Autodesk Inventor part; units mm, degrees
ref_plane "YZ Plane" through (0, 0, 0) normal (1, 0, 0) x (0, 1, 0)
ref_plane "XZ Plane" through (0, 0, 0) normal (0, 1, 0) x (-1, 0, 0)
ref_plane "XY Plane" through (0, 0, 0) normal (0, 0, 1) x (1, 0, 0)
sketch "Sketch1" plane through (0, 0, 0) normal (0, 1, 0) x (-1, 0, 0)
  line L0 (0, 0) -> (-34.29, 0)
  line L1 (-34.29, 0) -> (-34.29, 25.4)
  line L2 (-34.29, 25.4) -> (0, 25.4)
  line L3 (0, 25.4) -> (0, 0)
  line L4 (0, 25.4) -> (-2.54, 25.4) construction
  line L5 (-2.54, 25.4) -> (-2.54, 22.86) construction
  line L6 (-2.54, 22.86) -> (0, 22.86) construction
  line L7 (0, 22.86) -> (0, 25.4) construction
  line L8 (0, 0) -> (-2.54, 0) construction
  line L9 (-2.54, 0) -> (-2.54, 2.54) construction
  line L10 (-2.54, 2.54) -> (0, 2.54) construction
  line L11 (0, 2.54) -> (0, 0) construction
  line L12 (-34.29, 25.4) -> (-31.75, 25.4) construction
  line L13 (-31.75, 25.4) -> (-31.75, 22.86) construction
  line L14 (-31.75, 22.86) -> (-34.29, 22.86) construction
  line L15 (-34.29, 22.86) -> (-34.29, 25.4) construction
  line L16 (-34.29, 0) -> (-31.75, 0) construction
  line L17 (-31.75, 0) -> (-31.75, 2.54) construction
  line L18 (-31.75, 2.54) -> (-34.29, 2.54) construction
  line L19 (-34.29, 2.54) -> (-34.29, 0) construction
  circle A0 centre (-2.54, 22.86) radius 1.0922
  circle A1 centre (-2.54, 2.54) radius 1.0922
  circle A2 centre (-31.75, 2.54) radius 1.0922
  circle A3 centre (-31.75, 22.86) radius 1.0922
  line L20 (0.635, 26.035) -> (-34.925, 26.035)
  line L21 (-34.925, 26.035) -> (-34.925, -0.635)
  line L22 (-34.925, -0.635) -> (0.635, -0.635)
  line L23 (0.635, -0.635) -> (0.635, 26.035)
  dimension "d0" = 34.29
  dimension "d1" = 25.4
  dimension "d2" = 2.54
  dimension "d3" = 2.54
  dimension "d4" = 2.54
  dimension "d5" = 2.54
  dimension "d6" = 2.54
  dimension "d7" = 2.54
  dimension "d8" = 2.54
  dimension "d9" = 2.54
  dimension "d10" = 2.1844
  dimension "d11" = 2.1844
  dimension "d12" = 2.1844
  dimension "d13" = 2.1844
  dimension "d14" = 0.635
extrude "Extrusion1" add sketch "Sketch1" along normal blind 3.175 contours L0 L1 L2 L3 | L23 L22 L21 L20
sketch "Sketch2" plane through (0, 3.175, 0) normal (0, 1, 0) x (1, 0, 0)
  line L0 (34.925, -26.035) -> (34.925, 0.635)
  line L1 (34.925, 0.635) -> (-0.635, 0.635)
  line L2 (-0.635, 0.635) -> (-0.635, -26.035)
  line L3 (-0.635, -26.035) -> (34.925, -26.035)
  circle A0 centre (2.54, -22.86) radius 1.0922
  circle A1 centre (2.54, -2.54) radius 1.0922
  circle A2 centre (31.75, -2.54) radius 1.0922
  circle A3 centre (31.75, -22.86) radius 1.0922
  line L4 (-3.81, -29.21) -> (-3.81, 3.81)
  line L5 (-3.81, 3.81) -> (38.1, 3.81)
  line L6 (38.1, 3.81) -> (38.1, -29.21)
  line L7 (38.1, -29.21) -> (-3.81, -29.21)
  point P0 (0, 0)
  dimension "d17" = 3.175
extrude "Extrusion2" add sketch "Sketch2" along normal blind 24 and the other way blind 3.175 contours L4 L5 L6 L7
sketch "Sketch3" plane through (38.1, 0, -3.81) normal (1, 0, 0) x (0, 0, -1)
  line L0 (-3.175, 27.175) -> (-29.845, 27.175)
  line L1 (-16.51, 27.175) -> (-24.01, 27.175)
  line L2 (-24.01, 27.175) -> (-9.01, 27.175)
  line L3 (-9.01, 27.175) -> (-9.01, 3.175)
  line L4 (-29.845, 3.175) -> (-3.175, 3.175)
  line L5 (-24.01, 27.175) -> (-24.01, 3.175)
  point P0 (-3.81, 0)
  dimension "d22" = 7.5
  dimension "d23" = 15
extrude "Extrusion3" cut sketch "Sketch3" against normal blind 24
sketch "Sketch4" plane through (-0.635, 3.175, 26.035) normal (1, 0, 0) x (0, 0, -1)
  line L0 (29.845, 24) -> (-3.175, 24)
  line L1 (13.335, 24) -> (6.835, 24)
  line L2 (6.835, 24) -> (19.835, 24)
  line L3 (26.67, 0) -> (0, 0)
  line L4 (19.835, 24) -> (6.835, 24)
  line L5 (6.835, 24) -> (6.835, 0)
  line L6 (6.835, 0) -> (19.835, 0)
  line L7 (19.835, 0) -> (19.835, 24)
  point P0 (26.035, -3.175)
  dimension "d26" = 6.5
  dimension "d27" = 13
extrude "Extrusion4" cut sketch "Sketch4" against normal blind 24
sketch "Sketch5" plane through (0, 0, 0) normal (0, -1, 0) x (1, 0, 0)
  line L0 (38.1, -3.81) -> (38.1, 29.21)
  line L1 (38.1, 29.21) -> (-3.81, 29.21)
  line L2 (-3.81, 29.21) -> (-3.81, -3.81)
  line L3 (-3.81, -3.81) -> (38.1, -3.81)
  circle A0 centre (2.54, 22.86) radius 1.0922
  circle A1 centre (2.54, 2.54) radius 1.0922
  circle A2 centre (31.75, 2.54) radius 1.0922
  circle A3 centre (31.75, 22.86) radius 1.0922
  line L4 (-0.635, -0.635) -> (-0.635, 26.035)
  line L5 (-0.635, 26.035) -> (34.925, 26.035)
  line L6 (34.925, 26.035) -> (34.925, -0.635)
  line L7 (34.925, -0.635) -> (-0.635, -0.635)
  line L8 (17.145, 29.21) -> (17.145, 35.56)
  line L9 (17.145, -3.81) -> (17.145, -10.16)
  circle A4 centre (17.145, 35.56) radius 2
  circle A5 centre (17.145, -10.16) radius 2
  circle A6 centre (17.145, 35.56) radius 6.35
  circle A7 centre (17.145, -10.16) radius 6.35
  line L10 (23.495, 35.56) -> (23.495, 29.21)
  line L11 (10.795, 35.56) -> (10.795, 29.21)
  line L12 (10.795, -10.16) -> (10.795, -3.81)
  line L13 (23.495, -10.16) -> (23.495, -3.81)
  point P0 (0, 0)
  dimension "d30" = 3.175
  dimension "d31" = 6.35
  dimension "d32" = 6.35
  dimension "d33" = 4
  dimension "d34" = 4
extrude "Extrusion5" add sketch "Sketch5" along normal blind 6.35 contours L3 L2 L1 L0 | L13 A7 L3 | L1 A6 L10 | A7 L12 L3 | A7 | L1 L11 A6 | A6
sketch "Sketch6" plane through (0, 3.175, 0) normal (0, 1, 0) x (1, 0, 0)
  circle A0 centre (31.75, -22.86) radius 1.0922
  circle A1 centre (31.75, -2.54) radius 1.0922
  circle A2 centre (2.54, -2.54) radius 1.0922
  circle A3 centre (2.54, -22.86) radius 1.0922
  line L0 (34.925, -5.2) -> (34.925, 0.635)
  line L1 (34.925, 0.635) -> (-0.635, 0.635)
  line L2 (-0.635, 0.635) -> (-0.635, -6.2)
  line L3 (-0.635, -6.2) -> (-3.81, -6.2)
  line L4 (-3.81, -19.2) -> (-3.81, -6.2)
  line L5 (-0.635, -19.2) -> (-3.81, -19.2)
  line L6 (-0.635, -19.2) -> (-0.635, -26.035)
  line L7 (-0.635, -26.035) -> (34.925, -26.035)
  line L8 (34.925, -26.035) -> (34.925, -20.2)
  line L9 (38.1, -20.2) -> (34.925, -20.2)
  line L10 (38.1, -5.2) -> (38.1, -20.2)
  line L11 (38.1, -5.2) -> (34.925, -5.2)
  line L12 (-0.635, -6.2) -> (-0.635, -19.2)
  line L13 (34.925, -5.2) -> (34.925, -20.2)
  point P0 (0, 0)
extrude "Extrusion6" add sketch "Sketch6" along normal blind 4 contours L11 L10 L9 L13 | L12 L5 L4 L3
sketch "Sketch7" plane through (0, 0, 0) normal (0, 1, 0) x (1, 0, 0)
  line L0 (10.795, 3.81) -> (23.495, 3.81)
  line L1 (23.495, 10.16) -> (23.495, 3.81)
  arc A0 (23.495, 10.16) -> (10.795, 10.16) centre (17.145, 10.16) ccw
  line L2 (10.795, 3.81) -> (10.795, 10.16)
  circle A1 centre (17.145, 10.16) radius 2
  circle A2 centre (17.145, -35.56) radius 2
  line L3 (23.495, -29.21) -> (10.795, -29.21)
  line L4 (10.795, -35.56) -> (10.795, -29.21)
  arc A3 (10.795, -35.56) -> (23.495, -35.56) centre (17.145, -35.56) ccw
  line L5 (23.495, -29.21) -> (23.495, -35.56)
  point P0 (0, 0)
extrude "Extrusion7" cut sketch "Sketch7" against normal blind 3.175
properties part number "pololuCaseBottom"
The listing builds one solid part. Answer for the finished solid, in the listing's coordinates (mm). A direction names the side the tool comes from. Round coordinates to 2 decimals unless told otherwise and drop trailing zeros. Loops run counter-clockwise (first coordinate to the right, second up) from the corner with the lowest first, then second, coordinate; pieces in that order, holes last.
Q1. Find the intervals of material crossed by line 1 (Z direction, x = 6, y = 15.5) (3 decimals); line 2 (X direction, y = 11, z = 4) (3 decimals); line 3 (X direction, y = 2, z = 22), in increasing order.
Q2. Section A-A, the plane x = 2.54 is taken. Determine the outline of the cut face in (y, z) (3 decimals).
Q3. Which of the six approach directions +Z, -Z, +X, -X, +Y, -Y give full straight-line access (tool end or side, diameter ignored) to faces 1 (the face through (-2, 17, 19.2)), 2 (the face through (17, 15, 26.035)), 3 (the face through (23.495, -5, -7)), 4 (the face through (17, -3, -0.635))?
Q4. Section D-D, the plane x = 8.5 is taken. Determine the outline of the cut face in (y, z) (3 decimals).
Q5. For a pull along X with two mould halves and no side action, classify faces 5 (the face through (17, 0, 13)), 6 (the face through (10.795, -5, 32)), 7 (the face through (37, 17, 20.2)), 8 (the face through (38.1, 6, 12)) as released by +X, released by -X, zero draft, split by the parting line, or undercut.
Q6. Section C-C, the plane y = 5 is taken. Determine the outline of the cut face in (x, z) (3 decimals), then the cut area to 3 significant figures.
Q7. Given pin 1 Ø3.5 at (x, y) = (37, 17.5) entering from +Z; pin 2 Ø2 at (x, z) = (11.5, 18.5) entering from -Y; pin 3 Ø3.5 at (y, z) = (-5, 33) entering from +X (3 decimals), each flat-ended and moving along its own axis, determine where each tip first touches the part or whether it passes through.
Q8. Section B-B, the plane z = 0.5 is taken. Determine the outline of the cut face in (x, y) (3 decimals), then the cut area to 3 significant figures.
Completed:
1. line 1: z = -3.81 to -0.635, 26.035 to 29.21
1. line 2: x = -3.81 to -0.635, 34.925 to 38.1
1. line 3: x = -3.81 to 1.87, 3.21 to 31.08, 32.42 to 38.1
2. outline: (-6.35, -3.81) - (27.175, -3.81) - (27.175, -0.635) - (3.175, -0.635) - (3.175, 1.448) - (0, 1.448) - (0, -0.635) - (-6.35, -0.635) - close; (-6.35, 26.035) - (0, 26.035) - (0, 23.952) - (3.175, 23.952) - (3.175, 26.035) - (27.175, 26.035) - (27.175, 29.21) - (-6.35, 29.21) - close; (0, 3.632) - (3.175, 3.632) - (3.175, 21.768) - (0, 21.768) - close
3. face 1: +X, -X, +Y
3. face 2: +Y
3. face 3: -Z, +X, +Y, -Y
3. face 4: -Y
4. outline: (-6.35, -3.81) - (27.175, -3.81) - (27.175, -0.635) - (3.175, -0.635) - (3.175, 26.035) - (27.175, 26.035) - (27.175, 29.21) - (-6.35, 29.21) - (-6.35, 26.035) - (0, 26.035) - (0, -0.635) - (-6.35, -0.635) - close
5. face 5: undercut
5. face 6: released by -X
5. face 7: zero draft
5. face 8: released by +X
6. outline: (-3.81, -3.81) - (38.1, -3.81) - (38.1, 29.21) - (-3.81, 29.21) - close; hole (-0.635, -0.635) - (34.925, -0.635) - (34.925, 26.035) - (-0.635, 26.035) - close
6. area: 435 mm2
7. pin 1: stops at z = 29.21
7. pin 2: stops at y = 0
7. pin 3: stops at x = 23.495
8. outline: (-3.81, -6.35) - (-0.635, -6.35) - (-0.635, 0) - (34.925, 0) - (34.925, -6.35) - (38.1, -6.35) - (38.1, 27.175) - (34.925, 27.175) - (34.925, 3.175) - (-0.635, 3.175) - (-0.635, 27.175) - (-3.81, 27.175) - close
8. area: 326 mm2
